Design review of the part built by this model. Coordinates are the model's own, in mm. Face numbers are marked on the shaded views. A direction names the side the tool comes from. Give positions to 0.01 mm unless a question says otherwise; leave off trailing zeros. Order: outer loops, then holes, each group sorted by start corner. A loop starts at its lowest first (then second) coordinate and runs counter-clockwise, first axis right, second up. Notation, with made-up numbers: (80, 52.5) -> (95, 52.5) arc R17 cw to (95, 67.5) -> close; hole circle Ø6 at (-28.5, 46.5). An arc over 180 degrees is marked (long way). One line per item, written item: value. Start each with the question number.
1) Tool access review of the marked faces 1 and 2: name each direction out of +Z, -Z, +X, -X, +Y, -Y from which nothing blocks a thin tool from reaching the whole face with its end or side.
2) The part is to be moulded in two halves that separate along X. For the marked faces 3, 4 and 5, say which applies: released by +X, released by -X, zero draft, split by the parting line, or undercut.
3) Wall thickness on line 1 along X through (y, z) = (0.5, 18.5); line 2 along X through (y, z) = (3, 14.25); line 3 along Z through (x, y) = (-21, 3.5): over which ranges is each line inside the solid? List them lowest first. Write a range as from..to.
4) For pin 1 (1 mm diameter, centred on x = 11, z = 23, fed in from -Y); pin 2 (8 mm diameter, centred on x = -17.5, y = 1.5, fed in from +Z); pin 3 (8 mm diameter, centred on x = -19, y = 0.46, fed in from +Z), all flat-tipped, find the tip position at first contact; note any pin that passes through.
5) Consider section B-B (z = 9). State the section outline as (x, y) points.
6) Consider section A-A (x = -13). State the section outline as (y, z) points, plus the area to 3 significant figures.
from build123d import *

# Parameters (mm, degrees)
F0_W           = 73.618516326
F0_H           = 45.713365078
F1_DEPTH       = 25.4
F3_D           = 5.5
F3_CBORE_D     = 9.75
F3_CBORE_DEPTH = 5
F4_SIZE        = 5.08


with BuildPart() as f1:
    # F0 (on Top) → F1 (new body)
    with BuildSketch(Plane.XY):
        Rectangle(F0_W, F0_H)
    extrude(amount=F1_DEPTH)

    # F3 (through all)
    with Locations(Plane.XY.offset(25.4)):
        with Locations((0.0451991563, 0.4629576465), (-19.0048008437, 0.4629576465), (19.0951991563, 0.4629576465)):
            CounterBoreHole(F3_D / 2, F3_CBORE_D / 2, F3_CBORE_DEPTH)

    # F4
    f4_edges = [f1.edges().sort_by_distance(p)[0] for p in [
        (36.809258, 0, 25.4),
        (0, 22.856683, 25.4),
        (-36.809258, 0, 25.4),
        (0, -22.856683, 25.4),
    ]]
    chamfer(f4_edges, length=F4_SIZE)


solid = f1.part
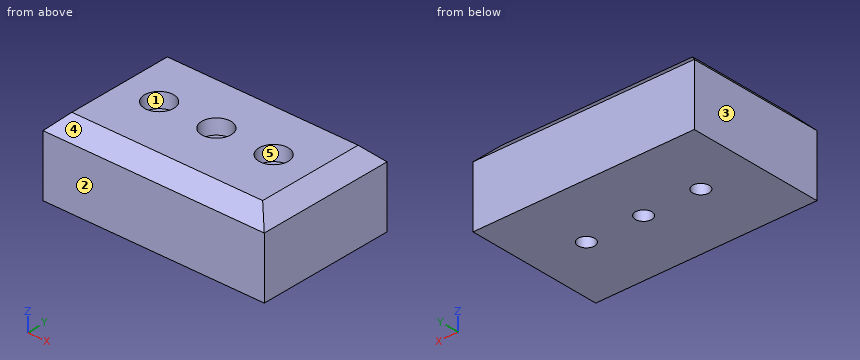
Checked values:
1. face 1: +Z
1. face 2: +Z, -Z, +X, -X, -Y
2. face 3: released by -X
2. face 4: zero draft
2. face 5: undercut
3. line 1: x = -36.81..-21.75, -16.26..-2.7, 2.79..16.35, 21.84..36.81
3. line 2: x = -36.81..-20.07, -17.94..-1.02, 1.11..18.03, 20.16..36.81
3. line 3: z = 0..20.4
4. pin 1: stops at y = -20.68
4. pin 2: stops at z = 25.4
4. pin 3: stops at z = 20.4
5. outline: (-36.81, -22.86) -> (36.81, -22.86) -> (36.81, 22.86) -> (-36.81, 22.86) -> close; hole circle Ø5.5 at (-19, 0.46); hole circle Ø5.5 at (0.05, 0.46); hole circle Ø5.5 at (19.1, 0.46)
6. outline: (-22.86, 0) -> (22.86, 0) -> (22.86, 20.32) -> (17.78, 25.4) -> (-17.78, 25.4) -> (-22.86, 20.32) -> close
6. area: 1,140 mm^2
